```python
from build123d import *

# Parameters (mm, degrees)
SKETCH024_R             = 2.1
POCKET008_DEPTH         = 8
POCKET015_DEPTH         = 14
BODY002_PLACEMENT_ANGLE = 325.1


with BuildPart() as part:
    # Sketch006 → Revolution001 (revolve)
    with BuildSketch(Plane.XZ):
        Polygon((37.6, 25), (39.2, 25), (44.894981, 12.787073), (51.557862, -25), (49.957862, -25), (49.252554, -21), (43.294981, -21), (43.294981, 12.787073), align=None)
    revolve(axis=Axis((0, 0, 0), (0, 0, 1)))

    # Sketch011 → AdditiveLoft section 0
    with BuildSketch(Plane.XY.offset(14)):
        with BuildLine():
            ThreePointArc((42.6105, 5.774535), (38.773466, 1.434698), (42.920734, -2.609704))
            ThreePointArc((42.920734, -2.609704), (42.970593, 1.59), (42.6105, 5.774535))
        make_face()
    # Sketch012 → AdditiveLoft section 1
    with BuildSketch(Plane(origin=(0, 1, 22), x_dir=(1, 0, 0), z_dir=(0, 0, 1))):
        with BuildLine():
            ThreePointArc((39.836792, 3.609708), (38.556329, 0.532049), (39.921227, -2.509107))
            ThreePointArc((39.921227, -2.509107), (39.996192, 0.551918), (39.836792, 3.609708))
        make_face()
    loft()

    # Sketch024 (on Face9 of AdditiveLoft) → Pocket008 (cut)
    with BuildSketch(Plane(origin=(0, 0, -21), x_dir=(1, 0, 0), z_dir=(0, 0, -1))):
        with Locations((-23.25, 40.270181)):
            Circle(SKETCH024_R)
        with Locations((46.5, 0)):
            Circle(SKETCH024_R)
        with Locations((-23.25, -40.270181)):
            Circle(SKETCH024_R)
    extrude(amount=-POCKET008_DEPTH, mode=Mode.SUBTRACT)

    # Sketch035 (on DatumPlane) → Pocket015 (cut)
    with BuildSketch(Plane(origin=(0, 194, 0), x_dir=(-0.258819, 0.965926, 0), z_dir=(0.965926, 0.258819, 0))):
        with BuildLine():
            ThreePointArc((-199.968301, 0.958611), (-200.675408, 0.665718), (-200.968301, -0.041389))
            Line((-200.968301, -5.041389), (-200.968301, -0.041389))
            ThreePointArc((-200.968301, -5.041389), (-200.675408, -5.748496), (-199.968301, -6.041389))
            Line((-189.968301, -6.041389), (-199.968301, -6.041389))
            ThreePointArc((-189.968301, -6.041389), (-189.261194, -5.748496), (-188.968301, -5.041389))
            Line((-188.968301, -0.041389), (-188.968301, -5.041389))
            ThreePointArc((-188.968301, -0.041389), (-189.261194, 0.665718), (-189.968301, 0.958611))
            Line((-199.968301, 0.958611), (-189.968301, 0.958611))
        make_face()
    extrude(amount=-POCKET015_DEPTH, mode=Mode.SUBTRACT)


with BuildPart() as part_1:
    # Body002 placement: moved
    add(part.part.rotate(Axis((0, 0, 0), (0, 0, -1)), BODY002_PLACEMENT_ANGLE))


solid = part_1.part
```
For this review, take the finished solid that the model builds, in its own axes (mm). A direction names the side the tool comes from. Coordinates: 2 decimals unless noted, no trailing zeros. Loops run counter-clockwise (first coordinate to the right, second up) from the corner with the lowest first, then second, coordinate; pieces in that order, holes last. Notation, with made-up numbers: (-9.5, 39.25) - (0.5, 39.25) arc R16 cw to (0.5, 60.25) - close; hole circle Ø8 at (2.25, -40). An arc over 180 degrees is marked (long way). Use one line per item in the form item = value. Start each with the question number.
1) Take a section at A-A (x = 0). State the section outline as (y, z) points.
2) Draft analysis for pull direction X (two halves, no side actions). For faces 6 (the face through (30.541, 33.375, 0.658)), 7 (the face through (-42.913, 5.741, -3.87)), 8 (the face through (-15, -35, 25)), state which applies: released by +X, released by -X, zero draft, split by the parting line, or undercut.
3) To check wall thickness, follow probe 1 along X at (y, z) = (0, -9); probe 2 along X at (y, z) = (28.5, 12.5); probe 3 along Y at (x, z) = (39.5, -13.5). State the ranges of each line that lie inside material, in increasing order. Write a range as from..to.
4) Take a section at C-C (z = -19.5). State the section outline as (x, y) points.
5) For pin 1 (10 mm diameter, centred on x = 34.5, y = 27.5, fed in from -Z); pin 2 (4 mm diameter, centred on x = 38.14, y = 26.6, fed in from -Z); pin 3 (2 mm diameter, centred on x = -21, z = -9.5, fed in from +Y), all flat-tipped, find the tip position at first contact; note any pin that passes through.
6) For faces 1 (the face through (30.89, 33.76, -5.76)), 2 (the face through (33, 25, 14)), 3 (the face through (28.563, 37.063, 2.026)), 4 (the face through (34, 29, 0.959)), 5 (the face through (38.49, 24.63, -2.58)), list the 3-axis set-ups (+Z, -Z, +X, -X, +Y, -Y) from which the entire face can be reached by the end or side of a thin tool; tool diameter is ignored.
From the geometry:
q1.outline = (-51.56, -25) - (-49.96, -25) - (-49.25, -21) - (-43.29, -21) - (-43.29, 12.79) - (-37.6, 25) - (-39.2, 25) - (-44.89, 12.79) - close; (37.6, 25) - (43.29, 12.79) - (43.29, -21) - (49.25, -21) - (49.96, -25) - (51.56, -25) - (44.89, 12.79) - (39.2, 25) - close
q2.face_6 = released by +X
q2.face_7 = undercut
q2.face_8 = zero draft
q3.probe_1 = -48.74..-43.29, 43.29..48.74
q3.probe_2 = -34.75..-32.59, 32.59..34.75
q3.probe_3 = -29.88..-17.73, 17.73..25.01, 28.2..29.88
q4.outline = circle Ø101.18 at (0, 0); hole circle Ø4.2 at (-42.11, 19.73); hole circle Ø86.59 at (0, 0); hole circle Ø4.2 at (3.97, -46.33); hole circle Ø4.2 at (38.14, 26.6)
q5.pin_1 = -21
q5.pin_2 = -13
q5.pin_3 = 44.58
q6.face_1 = +X
q6.face_2 = -Z
q6.face_3 = +Z
q6.face_4 = none
q6.face_5 = +Y
